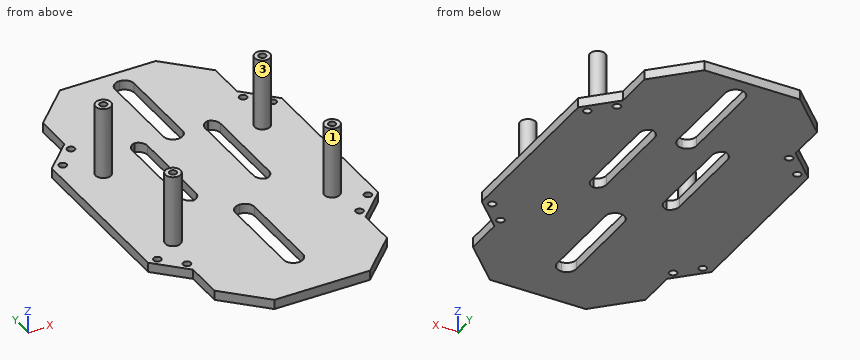
from build123d import *

# Parameters (mm, degrees)
ESQUISSE1_W             = 120
ESQUISSE1_H             = 120
BOSS_EXTRU_2_DEPTH      = 5
ESQUISSE9_R             = 4
BOSS_EXTRU_4_DEPTH      = 37.5
CHANFREIN5_SIZE         = 15
CHANFREIN6_SIZE         = 15
CHANFREIN7_SIZE         = 15
CHANFREIN8_SIZE         = 15
D_GAGEMENT_61_D         = 3.7973
D_GAGEMENT_61_DEPTH     = 10
D_GAGEMENT_61_TIP       = 1.140824014
ESQUISSE21_W            = 90
ESQUISSE21_H            = 5
BOSS_EXTRU_7_DEPTH      = 40
ESQUISSE22_W            = 90
ESQUISSE22_H            = 5
BOSS_EXTRU_8_DEPTH      = 40
CHANFREIN23_SIZE        = 20
ESQUISSE23_R            = 2
ENL_V_MAT_EXTRU_1_DEPTH = 10
SKETCH1_W               = 10
SKETCH1_H               = 55
CUT_EXTRUDE2_DEPTH      = 5
FILLET2_R               = 5
FILLET3_R               = 5
SKETCH3_W               = 10
SKETCH3_H               = 55
CUT_EXTRUDE4_DEPTH      = 5
FILLET11_R              = 5
SKETCH4_W               = 8
SKETCH4_H               = 55
CUT_EXTRUDE5_DEPTH      = 5
FILLET12_R              = 5
SKETCH4_2_W             = 8
SKETCH4_2_H             = 55
CUT_EXTRUDE6_DEPTH      = 5
FILLET16_R              = 5
FILLET17_R              = 5


# Some blends are built 0.0001 mm under size
with BuildPart() as part:
    # Esquisse1 → Boss.-Extru.2 (new body)
    with BuildSketch(Plane.XY):
        with Locations((18.92806479, -29.794391972)):
            Rectangle(ESQUISSE1_W, ESQUISSE1_H)
    extrude(amount=BOSS_EXTRU_2_DEPTH)

    # Esquisse9 → Boss.-Extru.4 (add)
    with BuildSketch(Plane.XY.offset(5)):
        with Locations(Location((-22.57193521, -64.794391972, 0), (0, 0, 180))):
            Circle(ESQUISSE9_R)
        with Locations(Location((-22.57193521, 0.205608028, 0), (0, 0, 180))):
            Circle(ESQUISSE9_R)
        with Locations(Location((60.42806479, 0.205608028, 0), (0, 0, 180))):
            Circle(ESQUISSE9_R)
        with Locations(Location((60.42806479, -64.794391972, 0), (0, 0, 180))):
            Circle(ESQUISSE9_R)
    extrude(amount=BOSS_EXTRU_4_DEPTH)

    # Chanfrein5
    chanfrein5_edges = [part.edges().sort_by_distance(p)[0] for p in [
        (78.92806479, -89.794391972, 2.5),
    ]]
    chamfer(chanfrein5_edges, length=CHANFREIN5_SIZE)

    # Chanfrein6
    chanfrein6_edges = [part.edges().sort_by_distance(p)[0] for p in [
        (78.92806479, 30.205608028, 2.5),
    ]]
    chamfer(chanfrein6_edges, length=CHANFREIN6_SIZE)

    # Chanfrein7
    chanfrein7_edges = [part.edges().sort_by_distance(p)[0] for p in [
        (-41.07193521, 30.205608028, 2.5),
    ]]
    chamfer(chanfrein7_edges, length=CHANFREIN7_SIZE)

    # Chanfrein8
    chanfrein8_edges = [part.edges().sort_by_distance(p)[0] for p in [
        (-41.07193521, -89.794391972, 2.5),
    ]]
    chamfer(chanfrein8_edges, length=CHANFREIN8_SIZE)

    # Dégagement #61
    with Locations(Plane(origin=(-22.57193521, -64.794391972, 42.5), x_dir=(1, 0, 0), z_dir=(0, 0, 1))):
        with Locations((0, 0), (83, 0), (83, 65), (0, 65)):
            Hole(D_GAGEMENT_61_D / 2, depth=D_GAGEMENT_61_DEPTH)
            with Locations((0, 0, -(D_GAGEMENT_61_DEPTH + D_GAGEMENT_61_TIP / 2))):  # 118° drill point
                Cone(0, D_GAGEMENT_61_D / 2, D_GAGEMENT_61_TIP, mode=Mode.SUBTRACT)

    # Esquisse21 → Boss.-Extru.7 (add)
    with BuildSketch(Plane(origin=(0, -89.794391972, 0), x_dir=(-1, 0, 0), z_dir=(0, -1, 0))):
        with Locations((-18.92806479, -2.5)):
            Rectangle(ESQUISSE21_W, ESQUISSE21_H)
    extrude(amount=BOSS_EXTRU_7_DEPTH)

    # Esquisse22 → Boss.-Extru.8 (add)
    with BuildSketch(Plane(origin=(0, 30.205608028, 0), x_dir=(1, 0, 0), z_dir=(0, 1, 0))):
        with Locations((18.92806479, -2.5)):
            Rectangle(ESQUISSE22_W, ESQUISSE22_H)
    extrude(amount=BOSS_EXTRU_8_DEPTH)

    # Chanfrein23
    chanfrein23_edges = [part.edges().sort_by_distance(p)[0] for p in [
        (-26.07193521, -129.794391972, 2.5),
        (63.92806479, -129.794391972, 2.5),
        (63.92806479, 70.205608028, 2.5),
        (-26.07193521, 70.205608028, 2.5),
    ]]
    chamfer(chanfrein23_edges, length=CHANFREIN23_SIZE)

    # Esquisse23 → Enlèv. mat.-Extru.1 (cut)
    with BuildSketch(Plane.XY.offset(5)):
        with Locations((-35.996277988, -74.213194945)):
            Circle(ESQUISSE23_R)
        with Locations((-26.096783051, -84.112689881)):
            Circle(ESQUISSE23_R)
        with Locations((-25.52408096, 25.096608028)):
            Circle(ESQUISSE23_R)
        with Locations((-35.390089468, 15.163739554)):
            Circle(ESQUISSE23_R)
        with Locations((63.953155144, 24.523663425)):
            Circle(ESQUISSE23_R)
        with Locations((73.85265008, 14.624168488)):
            Circle(ESQUISSE23_R)
        with Locations((63.953210541, -84.112391972)):
            Circle(ESQUISSE23_R)
        with Locations((73.852705477, -74.212897035)):
            Circle(ESQUISSE23_R)
    extrude(amount=-ENL_V_MAT_EXTRU_1_DEPTH, mode=Mode.SUBTRACT)

    # Sketch1 → Cut-Extrude2 (cut)
    with BuildSketch(Plane.XY.offset(5)):
        with Locations((18.92806479, -80.294391972)):
            Rectangle(SKETCH1_W, SKETCH1_H)
    extrude(amount=-CUT_EXTRUDE2_DEPTH, mode=Mode.SUBTRACT)

    # Fillet2
    fillet2_edges = [part.edges().sort_by_distance(p)[0] for p in [
        (13.92806479, -107.794391972, 2.5),
    ]]
    fillet(fillet2_edges, radius=FILLET2_R)

    # Fillet3
    fillet3_edges = [part.edges().sort_by_distance(p)[0] for p in [
        (13.92806479, -52.794391972, 2.5),
        (23.92806479, -52.794391972, 2.5),
        (23.92806479, -107.794391972, 2.5),
    ]]
    fillet(fillet3_edges, radius=FILLET3_R - 0.0001)  # a hair under: the kernel refuses the full size

    # Sketch3 → Cut-Extrude4 (cut)
    with BuildSketch(Plane.XY.offset(5)):
        with Locations((21.260912997, 36.166130895)):
            Rectangle(SKETCH3_W, SKETCH3_H)
    extrude(amount=-CUT_EXTRUDE4_DEPTH, mode=Mode.SUBTRACT)

    # Fillet11
    fillet11_edges = [part.edges().sort_by_distance(p)[0] for p in [
        (16.260912997, 63.666130895, 2.5),
        (26.260912997, 63.666130895, 2.5),
        (26.260912997, 8.666130895, 2.5),
        (16.260912997, 8.666130895, 2.5),
    ]]
    fillet(fillet11_edges, radius=FILLET11_R - 0.0001)  # a hair under: the kernel refuses the full size

    # Sketch4 → Cut-Extrude5 (cut)
    with BuildSketch(Plane.XY.offset(5)):
        with Locations((2.260912997, -12.123457497)):
            Rectangle(SKETCH4_W, SKETCH4_H)
        with Locations((40.260912997, -12.294391972)):
            Rectangle(SKETCH4_W, SKETCH4_H)
    extrude(amount=-CUT_EXTRUDE5_DEPTH, mode=Mode.SUBTRACT)

    # Fillet12
    # the kernel refuses this fillet: 5 mm, written as the material it adds along each edge
    with BuildSketch(Plane(origin=(44.260912997, 15.205608028, 5), x_dir=(0, -1, 0), z_dir=(0, 0, -1))) as fillet12_piece_1:
        with BuildLine():
            CenterArc((FILLET12_R, FILLET12_R), FILLET12_R, 180, 90)
            Line((0, FILLET12_R), (0, 0))
            Line((0, 0), (FILLET12_R, 0))
        make_face()
    extrude(amount=5)
    with BuildSketch(Plane(origin=(44.260912997, -39.794391972, 5), x_dir=(0, 1, 0), z_dir=(0, 0, -1)), Plane(origin=(36.260912997, 15.205608028, 5), x_dir=(0, -1, 0), z_dir=(0, 0, -1)), Plane(origin=(36.260912997, -39.794391972, 5), x_dir=(1, 0, 0), z_dir=(0, 0, -1))) as fillet12_piece_2:
        with BuildLine():
            CenterArc((FILLET12_R, -FILLET12_R), FILLET12_R, 90, 90)
            Line((0, -FILLET12_R), (0, 0))
            Line((0, 0), (FILLET12_R, 0))
        make_face()
    extrude(amount=5)

    # Sketch4<2> → Cut-Extrude6 (cut)
    with BuildSketch(Plane.XY.offset(5)):
        with Locations((2.260912997, -12.123457497)):
            Rectangle(SKETCH4_2_W, SKETCH4_2_H)
        with Locations((40.260912997, -12.294391972)):
            Rectangle(SKETCH4_2_W, SKETCH4_2_H)
    extrude(amount=-CUT_EXTRUDE6_DEPTH, mode=Mode.SUBTRACT)

    # Fillet16
    # the kernel refuses this fillet: 5 mm, written as the material it adds along each edge
    with BuildSketch(Plane(origin=(6.260912997, -39.623457497, 5), x_dir=(-1, 0, 0), z_dir=(0, 0, -1)), Plane(origin=(-1.739087003, 15.376542503, 5), x_dir=(1, 0, 0), z_dir=(0, 0, -1)), Plane(origin=(-1.739087003, -39.623457497, 5), x_dir=(0, 1, 0), z_dir=(0, 0, -1))) as fillet16_piece_1:
        with BuildLine():
            CenterArc((FILLET16_R, FILLET16_R), FILLET16_R, 180, 90)
            Line((0, FILLET16_R), (0, 0))
            Line((0, 0), (FILLET16_R, 0))
        make_face()
    extrude(amount=5)
    with BuildSketch(Plane(origin=(6.260912997, 15.376542503, 5), x_dir=(-1, 0, 0), z_dir=(0, 0, -1))) as fillet16_piece_2:
        with BuildLine():
            CenterArc((FILLET16_R, -FILLET16_R), FILLET16_R, 90, 90)
            Line((0, -FILLET16_R), (0, 0))
            Line((0, 0), (FILLET16_R, 0))
        make_face()
    extrude(amount=5)

    # Fillet17
    # the kernel refuses this fillet: 5 mm, written as the material it adds along each edge
    with BuildSketch(Plane(origin=(36.260912997, 15.205608028, 5), x_dir=(1, 0, 0), z_dir=(0, 0, -1)), Plane(origin=(36.260912997, -39.794391972, 5), x_dir=(0, 1, 0), z_dir=(0, 0, -1))) as fillet17_piece_1:
        with BuildLine():
            CenterArc((FILLET17_R, FILLET17_R), FILLET17_R, 180, 90)
            Line((0, FILLET17_R), (0, 0))
            Line((0, 0), (FILLET17_R, 0))
        make_face()
    extrude(amount=5)
    with BuildSketch(Plane(origin=(44.260912997, 15.205608028, 5), x_dir=(-1, 0, 0), z_dir=(0, 0, -1)), Plane(origin=(44.260912997, -39.794391972, 5), x_dir=(0, 1, 0), z_dir=(0, 0, -1))) as fillet17_piece_2:
        with BuildLine():
            CenterArc((FILLET17_R, -FILLET17_R), FILLET17_R, 90, 90)
            Line((0, -FILLET17_R), (0, 0))
            Line((0, 0), (FILLET17_R, 0))
        make_face()
    extrude(amount=5)


solid = part.part
For this review, take the finished solid that the model builds, in its own axes (mm). Face numbers are marked on the shaded views. Give positions to 0.01 mm unless a question says otherwise; leave off trailing zeros. Loops run counter-clockwise (first coordinate to the right, second up) from the corner with the lowest first, then second, coordinate; pieces in that order, holes last. Notation, with made-up numbers: M -18.5,21.25 L 33.5,21.25 A15 ccw 33.5,33.25 Z; hole C 24,-30 d9. An arc over 180 degrees is marked long. Put each result on its own line as item: value. Start each with the question number.
(1) Add section B-B, the plane z = 36.5. Write out the cut boundary in (x, y).
(2) Add section C-C, the plane y = -21.5. Write out the cut boundary in (x, z), then the cut area to 3 significant figures.
(3) The part is to be moulded in two halves that separate along Y. For the marked faces 1, 2 and 3, say which applies: +Y half, -Y half, draft (parallel to the pull), parting line (faces both ways), or undercut.
(4) For pin 1 (5.5 mm diameter, centred on y = -101.5, z = 3.5, fed in from +X); pin 2 (4 mm diameter, centred on x = 65.5, y = 46.5, fed in from +Z); pin 3 (5.5 mm diameter, centred on y = 40, z = 3.5, fed in from -X), all flat-tipped, find the tip position at first contact; note any pin that passes through.
(5) Wall thickness on L1, parallel to Z at x = 60, y = -26; L2, parallel to Y at x = -21.5, z = 19.5; L3, parallel to Y at x = 57, z = 21.5: over which ranges is each line inside the solid? List them lowest first.
(6) Add section A-A, the plane y = -99. Write out the cut boundary in (x, z), then the cut area to 3 significant figures.
(7) Add section D-D, the plane z = 12. Write out the cut boundary in (x, y).
Result:
1. outline: C -22.57,-64.79 d8; C -22.57,0.21 d8; C 60.43,-64.79 d8; C 60.43,0.21 d8; hole C -22.57,-64.79 d3.8; hole C -22.57,0.21 d3.8; hole C 60.43,-64.79 d3.8; hole C 60.43,0.21 d3.8
2. outline: M -41.07,0 L -1.74,0 L -1.74,5 L -41.07,5 Z; M 6.26,0 L 36.26,0 L 36.26,5 L 6.26,5 Z; M 44.26,0 L 78.93,0 L 78.93,5 L 44.26,5 Z
2. area: 520 mm^2
3. face 1: undercut
3. face 2: draft
3. face 3: undercut
4. pin 1: stops at x = 63.93
4. pin 2: stops at z = 5
4. pin 3: stops at x = -26.07
5. L1: z = 0 to 5
5. L2: y = -68.65 to -60.94, -3.65 to 4.06
5. L3: y = -66.86 to -62.73, -1.86 to 2.27
6. outline: M -26.07,0 L 13.93,0 L 13.93,5 L -26.07,5 Z; M 23.93,0 L 63.93,0 L 63.93,5 L 23.93,5 Z
6. area: 400 mm^2
7. outline: C -22.57,-64.79 d8; C -22.57,0.21 d8; C 60.43,-64.79 d8; C 60.43,0.21 d8
